```python
from build123d import *

# Parameters (mm, degrees)
SKETCH1_W           = 130.782832276
SKETCH1_H           = 75.259371088
SKETCH1_R           = 1.7
SKETCH1_R_2         = 7
SKETCH1_W_2         = 16.85151746
SKETCH1_H_2         = 19.689667769
SKETCH1_W_3         = 22.664698662
SKETCH1_H_3         = 16.485400984
BOSS_EXTRUDE3_DEPTH = 5
CUT_EXTRUDE1_DEPTH  = 3
FILLET1_R           = 2


with BuildPart() as part:
    # Sketch1 → Boss-Extrude3 (new body)
    with BuildSketch(Plane(origin=(0, 0, 0), x_dir=(1, 0, 0), z_dir=(0, 1, 0))):
        Rectangle(SKETCH1_W, SKETCH1_H)
        with Locations(Location((-58.42, 33.02, 0), (0, 0, 270))):
            Circle(SKETCH1_R, mode=Mode.SUBTRACT)
        with Locations(Location((-58.42, -33.02, 0), (0, 0, 270))):
            Circle(SKETCH1_R, mode=Mode.SUBTRACT)
        with Locations(Location((58.42, 33.02, 0), (0, 0, 270))):
            Circle(SKETCH1_R, mode=Mode.SUBTRACT)
        with Locations(Location((58.42, -33.02, 0), (0, 0, 270))):
            Circle(SKETCH1_R, mode=Mode.SUBTRACT)
        with Locations(Location((-20.838777713, 12.499959088, 0), (0, 0, 270))):
            Circle(SKETCH1_R, mode=Mode.SUBTRACT)
        with Locations(Location((-20.838777713, -12.500040912, 0), (0, 0, 270))):
            Circle(SKETCH1_R, mode=Mode.SUBTRACT)
        with Locations(Location((-9.838777713, 12.499959088, 0), (0, 0, 270))):
            Circle(SKETCH1_R, mode=Mode.SUBTRACT)
        with Locations(Location((-9.838777713, -12.500040912, 0), (0, 0, 270))):
            Circle(SKETCH1_R, mode=Mode.SUBTRACT)
        with Locations(Location((8.468303583, 12.485001846, 0), (0, 0, 270))):
            Circle(SKETCH1_R, mode=Mode.SUBTRACT)
        with Locations(Location((8.468303583, -9.090040912, 0), (0, 0, 270))):
            Circle(SKETCH1_R, mode=Mode.SUBTRACT)
        with Locations(Location((23.708296244, 12.499959088, 0), (0, 0, 270))):
            Circle(SKETCH1_R, mode=Mode.SUBTRACT)
        with Locations(Location((23.708296244, -9.090040912, 0), (0, 0, 270))):
            Circle(SKETCH1_R, mode=Mode.SUBTRACT)
        with Locations(Location((-47, 13, 0), (0, 0, 270))):
            Circle(SKETCH1_R, mode=Mode.SUBTRACT)
        with Locations(Location((-46.95213511, -13, 0), (0, 0, 270))):
            Circle(SKETCH1_R, mode=Mode.SUBTRACT)
        with Locations(Location((47, 13, 0), (0, 0, 270))):
            Circle(SKETCH1_R, mode=Mode.SUBTRACT)
        with Locations(Location((47, -13, 0), (0, 0, 270))):
            Circle(SKETCH1_R, mode=Mode.SUBTRACT)
        with Locations(Location((-49.48088922, 26.351150639, 0), (0, 0, 270))):
            Circle(SKETCH1_R_2, mode=Mode.SUBTRACT)
        with Locations(Location((-29.48088922, 26.351150639, 0), (0, 0, 270))):
            Circle(SKETCH1_R_2, mode=Mode.SUBTRACT)
        with Locations(Location((-9.48088922, 26.351150639, 0), (0, 0, 270))):
            Circle(SKETCH1_R_2, mode=Mode.SUBTRACT)
        with Locations(Location((10.51911078, 26.351150639, 0), (0, 0, 270))):
            Circle(SKETCH1_R_2, mode=Mode.SUBTRACT)
        with Locations(Location((30.51911078, 26.351150639, 0), (0, 0, 270))):
            Circle(SKETCH1_R_2, mode=Mode.SUBTRACT)
        with Locations(Location((50.51911078, 26.351150639, 0), (0, 0, 270))):
            Circle(SKETCH1_R_2, mode=Mode.SUBTRACT)
        with Locations(Location((-49.48088922, -26.480007122, 0), (0, 0, 270))):
            Circle(SKETCH1_R_2, mode=Mode.SUBTRACT)
        with Locations(Location((-29.48088922, -26.480007122, 0), (0, 0, 270))):
            Circle(SKETCH1_R_2, mode=Mode.SUBTRACT)
        with Locations(Location((-9.48088922, -26.480007122, 0), (0, 0, 270))):
            Circle(SKETCH1_R_2, mode=Mode.SUBTRACT)
        with Locations(Location((10.51911078, -26.480007122, 0), (0, 0, 270))):
            Circle(SKETCH1_R_2, mode=Mode.SUBTRACT)
        with Locations(Location((30.51911078, -26.480007122, 0), (0, 0, 270))):
            Circle(SKETCH1_R_2, mode=Mode.SUBTRACT)
        with Locations(Location((50.51911078, -26.480007122, 0), (0, 0, 270))):
            Circle(SKETCH1_R_2, mode=Mode.SUBTRACT)
        with Locations((-15.363894899, -0.098030908)):
            Rectangle(SKETCH1_W_2, SKETCH1_H_2, mode=Mode.SUBTRACT)
        with Locations((15.799758129, 1.504102484)):
            Rectangle(SKETCH1_W_3, SKETCH1_H_3, mode=Mode.SUBTRACT)
        with BuildLine():
            Line((-57.131435177, 5.386569447), (-32.131435177, 5.386569447))
            ThreePointArc((-32.131435177, 5.386569447), (-26.74486573, 0), (-32.131435177, -5.386569447))
            Line((-32.131435177, -5.386569447), (-57.131435177, -5.386569447))
            ThreePointArc((-57.131435177, -5.386569447), (-62.518004624, 0), (-57.131435177, 5.386569447))
        make_face(mode=Mode.SUBTRACT)
        with BuildLine():
            ThreePointArc((47.161472538, 3.408625582), (31.430083597, 1.352993065), (47.161472538, -0.702639453))
            ThreePointArc((47.161472538, -0.702639453), (62.892861479, 1.352993065), (47.161472538, 3.408625582))
        make_face(mode=Mode.SUBTRACT)
    extrude(amount=BOSS_EXTRUDE3_DEPTH)

    # Sketch2 → Cut-Extrude1 (cut)
    with BuildSketch(Plane.XZ):
        Polygon((-50.117691454, -13), (-48.558845727, -15.7), (-45.441154273, -15.7), (-43.882308546, -13), (-45.441154273, -10.3), (-48.558845727, -10.3), align=None)
        Polygon((-50.069826564, 13), (-48.510980837, 10.3), (-45.393289384, 10.3), (-43.834443657, 13), (-45.393289384, 15.7), (-48.510980837, 15.7), align=None)
        Polygon((43.882308546, -13), (45.441154273, -15.7), (48.558845727, -15.7), (50.117691454, -13), (48.558845727, -10.3), (45.441154273, -10.3), align=None)
        Polygon((43.882308546, 13), (45.441154273, 10.3), (48.558845727, 10.3), (50.117691454, 13), (48.558845727, 15.7), (45.441154273, 15.7), align=None)
    extrude(amount=-CUT_EXTRUDE1_DEPTH, mode=Mode.SUBTRACT)

    # Fillet1
    fillet1_edges = [part.edges().sort_by_distance(p)[0] for p in [
        (65.391416138, 2.5, 37.629685544),
        (-65.391416138, 2.5, 37.629685544),
        (-65.391416138, 2.5, -37.629685544),
        (65.391416138, 2.5, -37.629685544),
    ]]
    fillet(fillet1_edges, radius=FILLET1_R)


solid = part.part
```
The listing builds one solid part. Answer for the finished solid, in the listing's coordinates (mm). A direction names the side the tool comes from. Give positions to 0.01 mm unless a question says otherwise; leave off trailing zeros. Order: outer loops, then holes, each group sorted by start corner. A loop starts at its lowest first (then second) coordinate and runs counter-clockwise, first axis right, second up. Notation, with made-up numbers: (36, -28) -> (44, -28) arc R25 ccw to (44, -1) -> close; hole circle Ø9 at (-8, -24). An arc over 180 degrees is marked (long way). One line per item, written item: value.
1) A tool of negligible diameter and unlimited length cuts with its end or side. For faces 4 (the flat face through (-15, 2, -9.747)), 5 (the flat face through (47, 3, -11)), from which of +Z, -Z, +X, -X, +Y, -Y can it reach the whole face along a straight path? Write none if from no direction.
Reported:
face 4: +Y, -Y
face 5: -Y
2) Find the intervals of material crossed by line 1 (X direction, y = 4.1, z = 13); line 2 (Z direction, x = -18, y = 4.6); line 3 (X direction, y = 1.7, z = 10), in increasing order.
Reported:
line 1: x = -65.39 to -48.65, -45.25 to -22.46, -19.21 to -11.46, -8.21 to 45.3, 48.7 to 65.39
line 2: z = -37.63 to -9.75, 9.94 to 37.63
line 3: x = -65.39 to 7.03, 9.9 to 22.27, 25.14 to 65.39
3) Find section A-A, the plane x = 54. Determine the outline of the cut face in (y, z).
Reported:
outline: (0, -37.63) -> (5, -37.63) -> (5, -32.42) -> (0, -32.42) -> close; (0, -20.28) -> (5, -20.28) -> (5, -9.3) -> (0, -9.3) -> close; (0, 6.6) -> (5, 6.6) -> (5, 20.41) -> (0, 20.41) -> close; (0, 32.55) -> (5, 32.55) -> (5, 37.63) -> (0, 37.63) -> close
4) Find section C-C, the plane y = 1.55. Count the separate pieces of the cut face and the enclosed holes in it, plus the area to 3 significant figures.
Reported:
separate pieces: 1
enclosed holes: 32
area: 6,320 mm^2
5) Determine the mould class of faces 1 (the cylindrical face through (-59.07, 2.46, 34.59)), 2 (the cylindrical face through (45.5, 4, -12.2)), 3 (the flat face through (-1, 5, -1)) for opening direction X: pulls with the +X half, pulls with the -X half, needs draft (parallel to the pull), parting line crosses it, or undercut.
Reported:
face 1: undercut
face 2: undercut
face 3: needs draft
6) Find section B-B, the plane x = -15. Determine the outline of the cut face in (y, z).
Reported:
outline: (0, -37.63) -> (5, -37.63) -> (5, -30.66) -> (0, -30.66) -> close; (0, -22.05) -> (5, -22.05) -> (5, -9.75) -> (0, -9.75) -> close; (0, 9.94) -> (5, 9.94) -> (5, 22.17) -> (0, 22.17) -> close; (0, 30.79) -> (5, 30.79) -> (5, 37.63) -> (0, 37.63) -> close
